The model under review builds one solid part; all positions refer to its coordinate system, in mm. Face numbers are marked on the shaded views. A direction names the side the tool comes from. Give positions to 0.01 mm unless a question says otherwise; leave off trailing zeros. Order: outer loops, then holes, each group sorted by start corner. A loop starts at its lowest first (then second) coordinate and runs counter-clockwise, first axis right, second up.
```python
from build123d import *

# Parameters (mm, degrees)
SKETCH_1_W          = 26
SKETCH_1_H          = 26
SKETCH_1_R          = 10
EXTRUDE_1_DEPTH     = 5
CUT_EXTRUDE_START   = 0.5
CUT_EXTRUDE_3_DEPTH = 4


# Read off the part's stored shape, not the designer's step: 切除-拉伸3
with BuildPart() as part:
    # 草图1 → 凸台-拉伸1 (new body)
    with BuildSketch(Plane.XY):
        Rectangle(SKETCH_1_W, SKETCH_1_H)
        Circle(SKETCH_1_R, mode=Mode.SUBTRACT)
    extrude(amount=EXTRUDE_1_DEPTH)

    # 切除-拉伸3 outline → 切除-拉伸3 (cut)
    with BuildSketch(Plane.XY.offset(CUT_EXTRUDE_START)):
        with BuildLine():
            ThreePointArc((4.582575695, -10), (11, 0), (4.582575695, 10))
            Line((4.582575695, 10), (0, 10))
            ThreePointArc((0, 10), (10, 0), (0, -10))
            Line((0, -10), (4.582575695, -10))
        make_face()
        with BuildLine():
            ThreePointArc((0, -10), (-10, 0), (0, 10))
            Line((0, 10), (-4.582575695, 10))
            ThreePointArc((-4.582575695, 10), (-11, 0), (-4.582575695, -10))
            Line((-4.582575695, -10), (0, -10))
        make_face()
    extrude(amount=CUT_EXTRUDE_3_DEPTH, mode=Mode.SUBTRACT)


solid = part.part
```
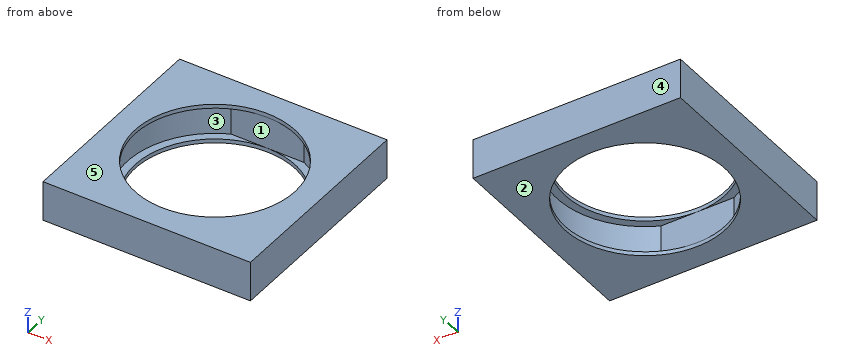
Item 1: For the marked faces 1 and 2, list the 3-axis set-ups (+Z, -Z, +X, -X, +Y, -Y) from which the entire face can be reached by the end or side of a thin tool; tool diameter is ignored.
Values found:
face 1: none
face 2: -Z, +X, -X, +Y, -Y
Item 2: Take a section at A-A (y = 0). Give the boundary of the cut face in (x, z), and give its area (3 significant figures).
Values found:
outline: (-13, 0) - (-10, 0) - (-10, 0.5) - (-11, 0.5) - (-11, 4.5) - (-10, 4.5) - (-10, 5) - (-13, 5) - close; (10, 0) - (13, 0) - (13, 5) - (10, 5) - (10, 4.5) - (11, 4.5) - (11, 0.5) - (10, 0.5) - close
area: 22.0 mm2
Item 3: Take a section at B-B (z = 4.15). Give the boundary of the cut face in (x, y), and give its area (3 significant figures).
Values found:
outline: (-13, -13) - (13, -13) - (13, 13) - (-13, 13) - close; hole (-4.58, -10) - (4.58, -10) arc R11 ccw to (4.58, 10) - (-4.58, 10) arc R11 ccw to start
area: 308 mm2
Item 4: For line 1 (Y direction, x = 0, z = 0.15); line 2 (Z direction, x = 5, y = -9), list the stretches that pass through material, from the lowest coordinate up.
Values found:
line 1: y = -13 to -10, 10 to 13
line 2: z = 0 to 0.5, 4.5 to 5
Item 5: Take a section at C-C (x = 1.75). Give the boundary of the cut face in (y, z), and give its area (3 significant figures).
Values found:
outline: (-13, 0) - (-9.85, 0) - (-9.85, 0.5) - (-10, 0.5) - (-10, 4.5) - (-9.85, 4.5) - (-9.85, 5) - (-13, 5) - close; (9.85, 0) - (13, 0) - (13, 5) - (9.85, 5) - (9.85, 4.5) - (10, 4.5) - (10, 0.5) - (9.85, 0.5) - close
area: 30.3 mm2
Item 6: Draft analysis for pull direction Y (two halves, no side actions). For the marked faces 3, 4 and 5, state which applies: released by +Y, released by -Y, zero draft, split by the parting line, or undercut.
Values found:
face 3: undercut
face 4: released by +Y
face 5: zero draft
